Answer from the drawing. Dimensions are ordinates in mm from the lowest x, y and z of the part. A direction names the side the tool comes from. Coordinates: 2 decimals unless noted, no trailing zeros. Loops run counter-clockwise (first coordinate to the right, second up) from the corner with the lowest first, then second, coordinate; pieces in that order, holes last. Notation, with made-up numbers: (85, 33) -> (139, 33) arc R20 cw to (139, 70) -> close; hole circle Ø8 at (-24.75, 34). An arc over 180 degrees is marked (long way). Answer as CSV lines item,"result".
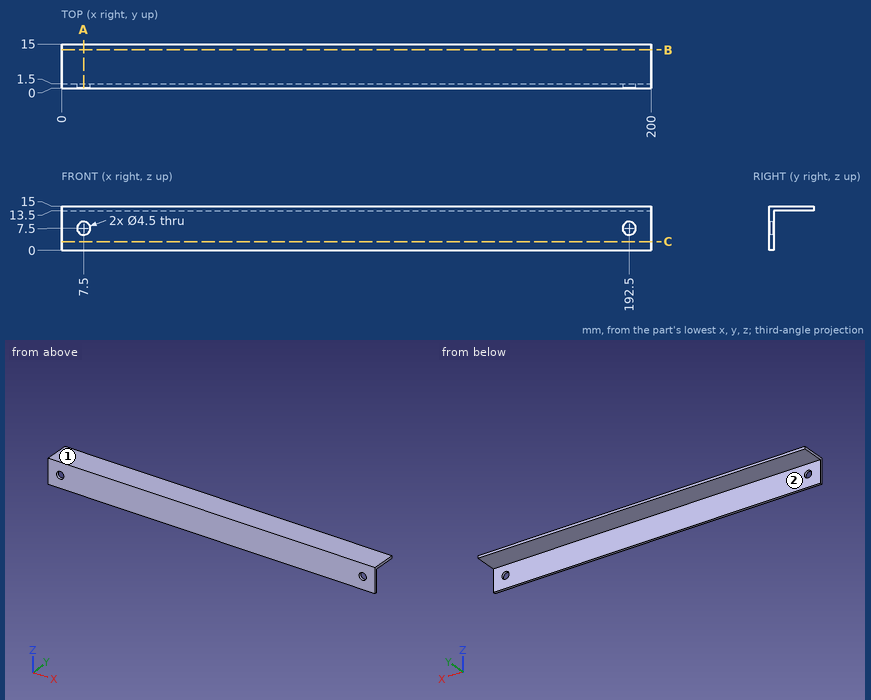
(1) Flat-ended cylindrical pins translate along their axes: pin 1 Ø1 at (x, z) = (76, 9) entering from +Y; pin 2 Ø4 at (x, y) = (52, 5.5) entering from -Z; pin 3 Ø4 at (x, z) = (192.5, 7.5) entering from +Y. Find the tip coordinate at first contact, or state that the pin passes through.
Computed values:
pin 1,"y = 1.5"
pin 2,"z = 13.5"
pin 3,"through"
(2) A cutting plane is placed at A-A, the plane x = 7.5. Write down the section's boundary in (y, z).
Computed values:
outline,"(0, 0) -> (1.5, 0) -> (1.5, 5.25) -> (0, 5.25) -> close; (0, 9.75) -> (1.5, 9.75) -> (1.5, 13.5) -> (15, 13.5) -> (15, 15) -> (0, 15) -> close"
(3) Consider line 1 along Z through (x, y) = (192.5, 0.7); line 2 along Z through (x, y) = (162.5, 12); line 3 along Y through (x, z) = (186, 1.75). Determine where each line is inside the solid, lowest interval first.
Computed values:
line 1,"0 to 5.25, 9.75 to 15"
line 2,"13.5 to 15"
line 3,"0 to 1.5"
(4) Which of the six approach directions +Z, -Z, +X, -X, +Y, -Y give full straight-line access (tool end or side, diameter ignored) to the marked faces 1 and 2?
Computed values:
face 1,"+Z, +X, -X, +Y, -Y"
face 2,"-Z, +X, -X, +Y"
(5) A cutting plane is placed at C-C, the plane z = 3. Write down the section's boundary in (x, y).
Computed values:
outline,"(0, 0) -> (200, 0) -> (200, 1.5) -> (0, 1.5) -> close"
(6) A cutting plane is placed at B-B, the plane y = 13. Write down the section's boundary in (x, z).
Computed values:
outline,"(0, 13.5) -> (200, 13.5) -> (200, 15) -> (0, 15) -> close"
